```python
from build123d import *

# Parameters (mm, degrees)
F0_R     = 15.875
F0_R_2   = 9.525
F1_DEPTH = 25.4
F2_DEPTH = 25.4
F3_DEPTH = 12.7
F4_R     = 6.35


with BuildPart() as f1:
    # F0 (on Top) → F1 (new body)
    with BuildSketch(Plane.XY):
        with BuildLine():
            ThreePointArc((8.2981181618, -27.3435890105), (22.9526616264, -17.0207505493), (28.575, 0))
            ThreePointArc((28.575, 0), (23.5615881585, 16.16731853), (10.2805336167, 26.6616063574))
            ThreePointArc((10.2805336167, 26.6616063574), (-28.5557674937, 1.0482212761), (8.2981181618, -27.3435890105))
        make_face()
        Circle(F0_R, mode=Mode.SUBTRACT)
        with BuildLine():
            ThreePointArc((69.85, 0), (64.2983142533, 13.442396078), (50.8790800715, 19.0498358613))
            ThreePointArc((50.8790800715, 19.0498358613), (31.7523183533, -0.2971933484), (51.4733508184, -19.0380959835))
            ThreePointArc((51.4733508184, -19.0380959835), (64.5063823289, -13.2301770001), (69.85, 0))
        make_face()
        with Locations((50.8, 0)):
            Circle(F0_R_2, mode=Mode.SUBTRACT)
        with BuildLine():
            ThreePointArc((10.2805336167, 26.6616063574), (23.5615881585, 16.16731853), (28.575, 0))
            ThreePointArc((28.575, 0), (22.9526616264, -17.0207505493), (8.2981181618, -27.3435890105))
            Line((8.2981181618, -27.3435890105), (51.4733508184, -19.0380959835))
            ThreePointArc((51.4733508184, -19.0380959835), (31.7523183533, -0.2971933484), (50.8790800715, 19.0498358613))
            Line((50.8790800715, 19.0498358613), (10.2805336167, 26.6616063574))
        make_face()
    extrude(amount=-F1_DEPTH)

    # F0 (on Top) → F2 (join)
    with BuildSketch(Plane.XY):
        with BuildLine():
            ThreePointArc((8.2981181618, -27.3435890105), (22.9526616264, -17.0207505493), (28.575, 0))
            ThreePointArc((28.575, 0), (23.5615881585, 16.16731853), (10.2805336167, 26.6616063574))
            ThreePointArc((10.2805336167, 26.6616063574), (-28.5557674937, 1.0482212761), (8.2981181618, -27.3435890105))
        make_face()
        Circle(F0_R, mode=Mode.SUBTRACT)
    extrude(amount=F2_DEPTH)

    # F0 (on Top) → F3 (cut)
    with BuildSketch(Plane.XY):
        with BuildLine():
            ThreePointArc((69.85, 0), (64.2983142533, 13.442396078), (50.8790800715, 19.0498358613))
            ThreePointArc((50.8790800715, 19.0498358613), (31.7523183533, -0.2971933484), (51.4733508184, -19.0380959835))
            ThreePointArc((51.4733508184, -19.0380959835), (64.5063823289, -13.2301770001), (69.85, 0))
        make_face()
        with Locations((50.8, 0)):
            Circle(F0_R_2, mode=Mode.SUBTRACT)
    extrude(amount=-F3_DEPTH, mode=Mode.SUBTRACT)

    # F4
    f4_edges = [f1.edges().sort_by_distance(p)[0] for p in [
        (51.473351, -19.038096, -6.35),
        (50.87908, 19.049836, -6.35),
    ]]
    fillet(f4_edges, radius=F4_R)


solid = f1.part
```
Could you check a few things on this model? Use its own coordinates, in mm. A direction names the side the tool comes from. Give positions to 0.01 mm unless a question says otherwise; leave off trailing zeros. Loops run counter-clockwise (first coordinate to the right, second up) from the corner with the lowest first, then second, coordinate; pieces in that order, holes last. Notation, with made-up numbers: (7.25, 60) - (18.25, 60) arc R23 cw to (18.25, 82) - close; hole circle Ø3 at (51.25, 51). An arc over 180 degrees is marked (long way). Use one line per item in the form item = value.
1. Thinking about a two-plate mould opening in Y: for faces 1 (the face through (26.35, 23.65, -15.34)), 2 (the face through (59.6, -3.65, -18.96)), 3 (the face through (20, 0, -25.4)), 4 (the face through (-3.441, -15.497, -0.356)), which applies, released by +Y, released by -Y, zero draft, split by the parting line, or undercut?
Response values:
face_1 = released by +Y
face_2 = undercut
face_3 = zero draft
face_4 = undercut
2. I want a section at B-B (z = 22.5). Please give me the cut outline in (x, y) (3 decimals), and give its area (3 significant figures).
Response values:
outline = circle Ø57.15 at (0, 0); hole circle Ø31.75 at (0, 0)
area = 1,770 mm²
3. On a 3-axis mill with a long thin cutter (end or side, diameter ignored), from which of +Z, -Z, +X, -X, +Y, -Y can I reach the whole of each face in a straight line? I mean faces 5 (the face through (37.23, 18.5, -6.44)), 6 (the face through (12, -12, 25.4)). Say none if no direction works.
Response values:
face_5 = +Z, +X
face_6 = +Z, +X, -X, +Y, -Y
4. I want a section at D-D (y = -17.5). Please give me the cut outline in (x, z), and give its area (3 significant figures).
Response values:
outline = (-22.59, -25.4) - (58.33, -25.4) - (58.33, -12.7) - (37.69, -12.7) - (37.69, 0) - (22.59, 0) - (22.59, 25.4) - (-22.59, 25.4) - close
area = 2,940 mm²
5. I want a section at A-A (x = 0). Please give me the cut outline in (y, z) (3 decimals).
Response values:
outline = (-28.575, -25.4) - (-15.875, -25.4) - (-15.875, 25.4) - (-28.575, 25.4) - close; (15.875, -25.4) - (28.575, -25.4) - (28.575, 25.4) - (15.875, 25.4) - close
6. I'm going to push flat-ended pins straight in: pin 1 Ø1 at (y, z) = (-1.5, -9.5) entering from -X; pin 2 Ø4 at (x, z) = (-13, 7) entering from +Y; pin 3 Ø8 at (x, y) = (-14, -0.5) entering from +Z; pin 4 Ø2 at (x, z) = (-12.5, -7.5) entering from -Y. Where does each tip first touch, or does it pass through?
Response values:
pin_1 = -28.56
pin_2 = 26.37
pin_3 = 25.4
pin_4 = -26.16
7. I need wall thicknesses on probe 1 along Y at (x, z) = (0, -10) (3 decimals); probe 2 along X at (y, z) = (0.5, -12.5); probe 3 along X at (y, z) = (-7.5, -23). Which ranges of each line are inside material? Lowest first, please.
Response values:
probe_1 = -28.575 to -15.875, 15.875 to 28.575
probe_2 = -28.57 to -15.87, 15.87 to 31.76
probe_3 = -27.57 to -13.99, 13.99 to 44.93, 56.67 to 68.31
8. I want a section at C-C (y = -1). Please give me the cut outline in (x, z), and give its area (3 significant figures).
Response values:
outline = (-28.56, -25.4) - (-15.84, -25.4) - (-15.84, 25.4) - (-28.56, 25.4) - close; (15.84, -25.4) - (41.33, -25.4) - (41.33, -12.7) - (31.78, -12.7) - (31.78, 0) - (28.56, 0) - (28.56, 25.4) - (15.84, 25.4) - close; (60.27, -25.4) - (69.82, -25.4) - (69.82, -12.7) - (60.27, -12.7) - close
area = 1,620 mm²
